Geometry: see drawing. Coordinates: mm, zero at the bounding-box minimum. Round coordinates to 2 decimals unless told otherwise and drop trailing zeros. Loops run counter-clockwise (first coordinate to the right, second up) from the corner with the lowest first, then second, coordinate; pieces in that order, holes last. Notation, with made-up numbers: (42.5, 5.25) - (89.5, 5.25) arc R17 ccw to (89.5, 23.25) - close; hole circle Ø9 at (55.25, -36). An arc over 180 degrees is marked (long way). Return JSON: item names as keys, results as strings. Group by question number.
1. Section B-B on z = 127. Return loops of the section in (x, y), and give its area (3 significant figures).
2. Material intervals for probe 1 along X at (y, z) = (7, 127); probe 2 along Z at (x, y) = (69, 5.5); probe 3 along Z at (x, y) = (58.5, 1.25), sorted ascending.
3. Section A-A on x = 63.5. Return loops of the section in (y, z), and give its area (3 significant figures).
4. Section C-C on y = 9. Return loops of the section in (x, z) (1 decimal).
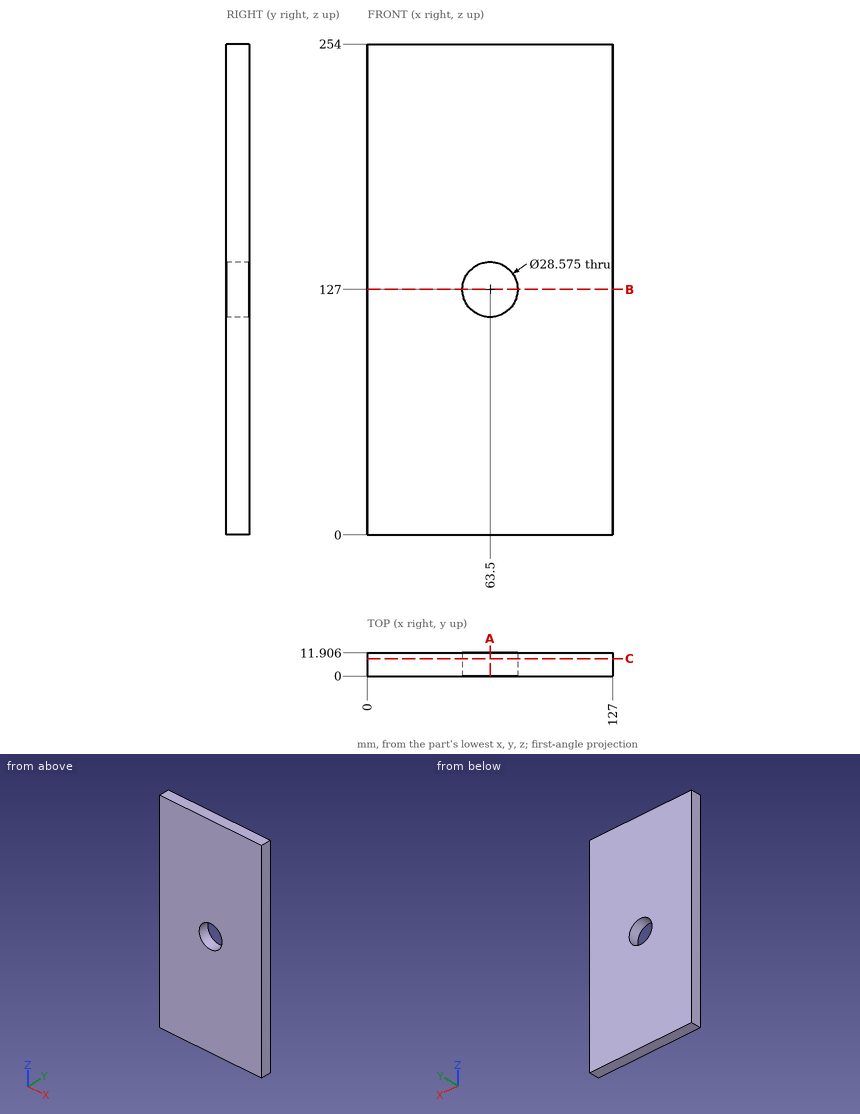
Taken from the geometry:
{
 "1": {"outline": "(0, 0) - (49.21, 0) - (49.21, 11.91) - (0, 11.91) - close; (77.79, 0) - (127, 0) - (127, 11.91) - (77.79, 11.91) - close", "area": "1,170 mm2"},
 "2": {"probe 1": "0 to 49.21, 77.79 to 127", "probe 2": "0 to 113.81, 140.19 to 254", "probe 3": "0 to 113.62, 140.38 to 254"},
 "3": {"outline": "(0, 0) - (11.91, 0) - (11.91, 112.71) - (0, 112.71) - close; (0, 141.29) - (11.91, 141.29) - (11.91, 254) - (0, 254) - close", "area": "2,680 mm2"},
 "4": {"outline": "(0, 0) - (127, 0) - (127, 254) - (0, 254) - close; hole circle Ø28.6 at (63.5, 127)"}
}
